from build123d import *

# Parameters (mm, degrees)
F0_R     = 5
F0_R_2   = 1
F1_DEPTH = 1.5
F2_R     = 2
F2_R_2   = 1
F3_DEPTH = 3.8
F4_R     = 0.6498381819
F5_DEPTH = 1.5


# Not quite as in the source:
# - a feature names something its author has since deleted; it is built from what else it names


with BuildPart() as f1:
    # F0 (on Top) → F1 (new body)
    with BuildSketch(Plane.XY):
        Circle(F0_R)
        Circle(F0_R_2, mode=Mode.SUBTRACT)
    extrude(amount=F1_DEPTH)

    # F2 (on face) → F3 (join)
    with BuildSketch(Plane.XY.offset(1.5)):
        Circle(F2_R)
        Circle(F2_R_2, mode=Mode.SUBTRACT)
    extrude(amount=F3_DEPTH)

    # F4 (on Top) → F5 (cut, through all)
    with BuildSketch(Plane.XY):
        with Locations((0, -3.5616646055)):
            Circle(F4_R)
    extrude(amount=F5_DEPTH, mode=Mode.SUBTRACT)


solid = f1.part
Part model, mm, in its own coordinate system. Coordinates: 2 decimals unless noted, no trailing zeros. Loops run counter-clockwise (first coordinate to the right, second up) from the corner with the lowest first, then second, coordinate; pieces in that order, holes last. Notation, with made-up numbers: (-2, 45.25) -> (47, 45.25) arc R12 cw to (47, 65.25) -> close; hole circle Ø4 at (73.5, -17). An arc over 180 degrees is marked (long way). Use a Markdown table: item, result. Add a question column.
Item 1: Pull direction Y, two halves, no side cores. Call faces 1 (the flat face through (2.2, 0.1, 1.5)), 2 (the cylindrical face through (0, -1, 3)), 3 (the cylindrical face through (0, -2, 3)): +Y half, -Y half, draft (parallel to the pull), parting line (faces both ways), or undercut.
Item 2: Band-saw the part on B-B on x = 0. Write the cut outline in (y, z).
Item 3: Band-saw the part on D-D on y = 3. Write the cut outline in (x, z), plus the area to 3 significant figures.
Item 4: Probe probe 1 along Y at (x, z) = (0, 1.15); probe 2 along Y at (x, z) = (0, 1.8); probe 3 along Z at (x, y) = (-2.5, 2.5). List the from-to ranges inside material, lowest first.
Item 5: Flat gauge pins, fed straight in: P1, Ø3, axis at y = 2, z = 4.5, coming from the -X side; P2, Ø1.5, axis at x = 2.5, z = 1.5, coming from the -Y side; P3, Ø1.5, axis at x = 0, y = -3.56, coming from the +Z side. Where does each tip first touch, or does it go through?
Item 6: Band-saw the part on A-A on y = 0. Write the cut outline in (x, z), plus the area to 3 significant figures.
Item 7: Band-saw the part on C-C on z = 3.4. Write the cut outline in (x, y).
Geometry says:
| question | item | result |
|---|---|---|
| 1 | face 1 | draft |
| 1 | face 2 | undercut |
| 1 | face 3 | parting line |
| 2 | outline | (-5, 0) -> (-4.21, 0) -> (-4.21, 1.5) -> (-5, 1.5) -> close; (-2.91, 0) -> (-1, 0) -> (-1, 5.3) -> (-2, 5.3) -> (-2, 1.5) -> (-2.91, 1.5) -> close; (1, 0) -> (5, 0) -> (5, 1.5) -> (2, 1.5) -> (2, 5.3) -> (1, 5.3) -> close |
| 3 | outline | (-4, 0) -> (4, 0) -> (4, 1.5) -> (-4, 1.5) -> close |
| 3 | area | 12.0 mm² |
| 4 | probe 1 | -5 to -4.21, -2.91 to -1, 1 to 5 |
| 4 | probe 2 | -2 to -1, 1 to 2 |
| 4 | probe 3 | 0 to 1.5 |
| 5 | P1 | x = -1.94 |
| 5 | P2 | y = -4.68 |
| 5 | P3 | z = 1.5 |
| 6 | outline | (-5, 0) -> (-1, 0) -> (-1, 5.3) -> (-2, 5.3) -> (-2, 1.5) -> (-5, 1.5) -> close; (1, 0) -> (5, 0) -> (5, 1.5) -> (2, 1.5) -> (2, 5.3) -> (1, 5.3) -> close |
| 6 | area | 19.6 mm² |
| 7 | outline | circle Ø4 at (0, 0); hole circle Ø2 at (0, 0) |
